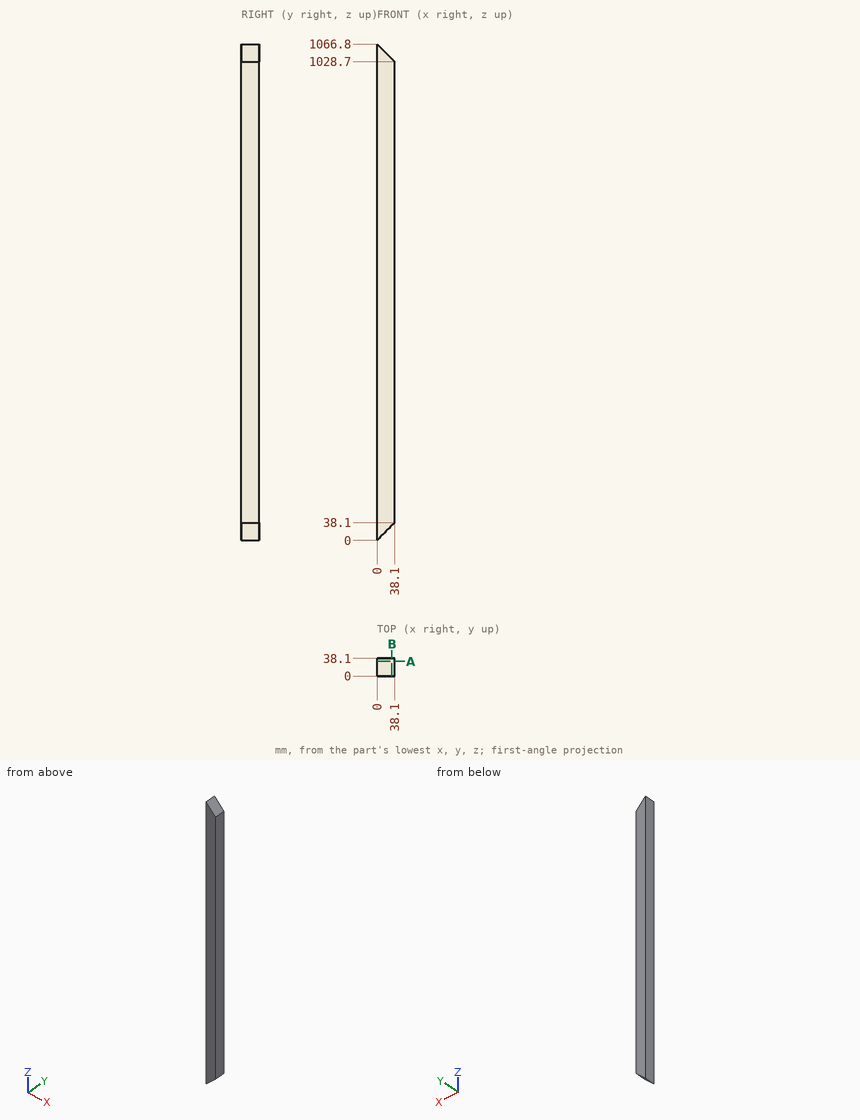
Geometry check sheet. Reference: drawing and pictorial views, mm from the part's lowest x, y, z. Give positions to 0.01 mm unless a question says otherwise; leave off trailing zeros. Loops run counter-clockwise (first coordinate to the right, second up) from the corner with the lowest first, then second, coordinate; pieces in that order, holes last. Notation, with made-up numbers: (-16, 65) -> (-10, 65) arc R23 cw to (-10, 92) -> close; hole circle Ø2 at (-35.5, 3.5). An arc over 180 degrees is marked (long way). Answer in a Markdown table with one row per item. Add a question column.
1) Cross-section at A-A on y = 31.5. Record the boundary of the cut face in (x, z).
2) Gauge pin test, flat ends, axial feed: P1, Ø3, axis at x = 18.5, y = 13, coming from the -Z side; P2, Ø10, axis at y = 26, z = 179, coming from the -X side; P3, Ø1.5, axis at x = 6.5, y = 5.5, coming from the -Z side; P4, Ø10, axis at x = 12, y = 23, coming from the -Z side. Record the tip position at first contact, or that the pin passes through.
3) Cross-section at B-B on x = 32. Record the boundary of the cut face in (y, z), and give its area (3 significant figures).
4) Material ranges on probe 1 along Z at (x, y) = (24, 25); probe 2 along Z at (x, y) = (32.5, 25), recorded low to high. Write a range as from..to.
Outcome:
| question | item | result |
|---|---|---|
| 1 | outline | (0, 0) -> (38.1, 38.1) -> (38.1, 1028.7) -> (0, 1066.8) -> close |
| 2 | P1 | stops at z = 17 |
| 2 | P2 | stops at x = 0 |
| 2 | P3 | stops at z = 5.75 |
| 2 | P4 | stops at z = 7 |
| 3 | outline | (0, 32) -> (38.1, 32) -> (38.1, 1034.8) -> (0, 1034.8) -> close |
| 3 | area | 38,200 mm^2 |
| 4 | probe 1 | z = 24..1042.8 |
| 4 | probe 2 | z = 32.5..1034.3 |
